Geometry: final body of the model. Coordinates: model frame, mm. Face numbers are marked on the shaded views. A direction names the side the tool comes from. Give positions to 0.01 mm unless a question says otherwise; leave off trailing zeros. Write each loop counter-clockwise with the first axis right and the second up, starting at its lowest first coordinate (ties: lowest second). Pieces come first, ordered by that corner, then holes. Notation, with made-up numbers: (82, 82) - (122, 82) arc R16 ccw to (122, 112) - close; hole circle Ø8 at (-30, -18). An arc over 180 degrees is marked (long way). Use CSV: the item, a comma, the result in double quotes. Start each with the question number.
(1) Section B-B on z = 3. Output: boundary loops of the cut face in (x, y), and give its area (3 significant figures).
(2) Line query: probe 1 along Z at (x, y) = (3.75, 9.5); probe 2 along X at (y, z) = (14, 7); probe 3 along X at (y, z) = (12, 9.75). Output: solid intervals per line, ascending. Write a range as [from, to].
(3) Section A-A on y = 7. Output: boundary loops of the cut face in (x, z).
(4) Section D-D on x = 16.5. Output: boundary loops of the cut face in (y, z).
(5) Reachability of the marked faces 4 and 5 from +Z, -Z, +X, -X, +Y, -Y: full face, straight path, thin tool, end or side. Return the list, or none.
(6) Draft query along X for the marked faces 1, 2 and 3. Return one class per face: released by +X, released by -X, zero draft, split by the parting line, or undercut.
(7) Section C-C on y = 14. Output: boundary loops of the cut face in (x, z), and give its area (3 significant figures).
(8) First-contact query: pin 1 Ø6 at (x, y) = (10.5, 39.5) entering from -Z; pin 2 Ø6 at (x, z) = (16, 4.5) entering from +Y; pin 3 Ø3 at (x, z) = (4, 5) entering from -Y; pin 4 Ø3 at (y, z) = (7, 4) entering from +X. Flat tips, straight axial feed; report the tip coordinate or a pass-through.
from build123d import *

# Parameters (mm, degrees)
F1_DEPTH = 10
F2_SIZE  = 1
F3_W     = 5.5
F3_H     = 5.5
F4_DEPTH = 10


with BuildPart() as f1:
    # F0 (on Top) → F1 (new body)
    with BuildSketch(Plane.XY):
        Polygon((0, 50), (0, 0), (7.5, 0), (7.5, 20), (17.5, 0), (25, 0), align=None)
    extrude(amount=F1_DEPTH)

    # F2
    f2_edges = [f1.edges().sort_by_distance(p)[0] for p in [
        (12.5, 10, 10),
        (7.5, 10, 10),
        (0, 25, 10),
        (12.5, 25, 10),
        (12.5, 10, 0),
        (7.5, 10, 0),
        (0, 25, 0),
        (12.5, 25, 0),
    ]]
    chamfer(f2_edges, length=F2_SIZE)

    # F3 (on face) → F4 (cut)
    with BuildSketch(Plane.XZ):
        with Locations((3.75, 5)):
            Rectangle(F3_W, F3_H)
    extrude(amount=-F4_DEPTH, mode=Mode.SUBTRACT)


solid = f1.part
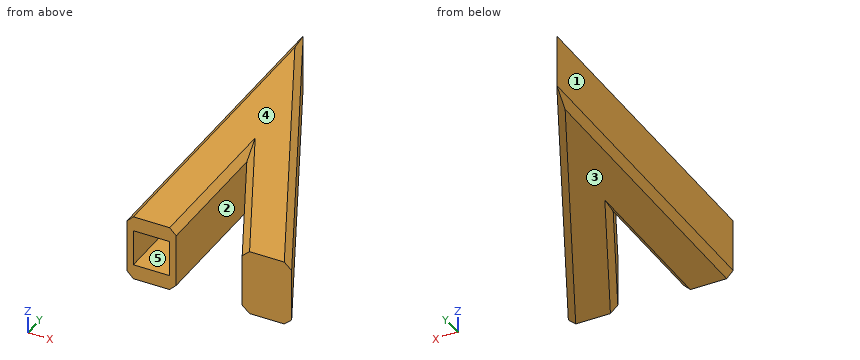
Check values:
1,outline,"(0, 0) - (1, 0) - (1, 10) - (6.5, 10) - (6.5, 0) - (7.5, 0) - (7.5, 20) - (17.5, 0) - (25, 0) - (0, 50) - close"
1,area,"470 mm²"
2,probe 1,"z = [0, 2.25], [7.75, 10]"
2,probe 2,"x = [0, 7.5], [10.5, 18]"
2,probe 3,"x = [0.75, 6.75], [12.34, 18.16]"
3,outline,"(0, 1) - (1, 0) - (6.5, 0) - (7.5, 1) - (7.5, 9) - (6.5, 10) - (1, 10) - (0, 9) - close; (14, 1) - (15.12, 0) - (20.38, 0) - (21.5, 1) - (21.5, 9) - (20.38, 10) - (15.12, 10) - (14, 9) - close; hole (1, 2.25) - (6.5, 2.25) - (6.5, 7.75) - (1, 7.75) - close"
4,outline,"(2, 1) - (4.24, 0) - (14.76, 0) - (17, 1) - (17, 9) - (14.76, 10) - (4.24, 10) - (2, 9) - close"
5,face 4,"+Z, +X, -X, +Y, -Y"
5,face 5,"-Y"
6,face 1,"released by -X"
6,face 2,"undercut"
6,face 3,"zero draft"
7,outline,"(0, 1) - (1, 0) - (6.5, 0) - (7.5, 1) - (7.5, 9) - (6.5, 10) - (1, 10) - (0, 9) - close; (10.5, 1) - (11.62, 0) - (16.88, 0) - (18, 1) - (18, 9) - (16.88, 10) - (11.62, 10) - (10.5, 9) - close"
7,area,"146 mm²"
8,pin 1,"passes through"
8,pin 2,"stops at y = 24"
8,pin 3,"stops at y = 10"
8,pin 4,"stops at x = 22.25"
